Autodesk Fusion 360 part; units mm, degrees
sketch "Sketch1" plane through (0, 0, 0) normal (0, 1, 0) x (1, 0, 0)
  line L0 (16, 0) -> (16, 35)
  line L1 (28.7, 0) -> (28.7, 35)
  line L2 (16, 35) -> (11, 35)
  line L3 (11, 35) -> (11, 0)
  line L4 (16, 0) -> (28.7, 0)
  line L5 (28.7, 35) -> (33.7, 35)
  line L6 (33.7, 35) -> (33.7, 0)
  line L7 (33.7, 0) -> (63.7, 0)
  line L8 (63.7, 0) -> (63.7, -10)
  line L9 (11, 0) -> (-19, 0)
  line L10 (-19, 0) -> (-19, -10)
  line L11 (-19, -10) -> (63.7, -10)
  dimension "d2" = 12.7
  dimension "d3" = 5
  dimension "d4" = 5
  dimension "d5" = 30
  dimension "d6" = 10
  dimension "d7" = 30
  dimension "d8" = 10
  dimension "d16" = 35
extrude "Extrude1" add sketch "Sketch1" along normal blind 35
sketch "Sketch2" plane through (33.7, 0, 0) normal (1, 0, 0) x (0, 0, -1)
  line L0 (0, 0) -> (35, 0)
  line L1 (35, 0) -> (35, 35)
  line L2 (35, 35) -> (0, 35)
  line L3 (0, 35) -> (0, 0)
  circle A0 centre (17.9261, 17.0739) radius 2.25
  line L4 (0, 35) -> (16.3351, 18.6649)
  line L5 (19.5171, 15.4829) -> (35, 0)
  line L6 (35, 35) -> (19.0329, 19.0329)
  line L7 (15.9671, 15.9671) -> (0, 0)
  dimension "d11" = 4.5
extrude "Extrude2" cut sketch "Sketch2" against normal blind 59 contours A0
ref_plane "WorkPlane1" through (22.35, 17.5, -12.5) normal (0, 1, 0) x (0, 0, 1)
sketch "Sketch3" plane through (0, 17.5, 0) normal (0, 1, 0) x (1, 0, 0)
  line L0 (-20, 0) -> (5, 0)
  line L1 (5, 0) -> (5, -10)
  line L2 (5, -10) -> (-20, -10)
  line L3 (-20, -10) -> (-20, 0)
  line L4 (44, 0) -> (44.05, 0)
  line L5 (33.7, 0) -> (33.7, 35)
  dimension "d14" = 25
sketch "Sketch4" plane through (11, 0, 0) normal (-1, 0, 0) x (0, 0, 1)
  circle A0 centre (-17.9261, 17.0739) radius 2.25 construction
  line L0 (-35, 0) -> (0, 0)
  line L1 (0, 0) -> (0, 35)
  line L2 (0, 35) -> (-35, 35)
  line L3 (-35, 35) -> (-35, 0)
  line L4 (-15.8332, 13.4489) -> (-13.7403, 17.0739)
  line L5 (-13.7403, 17.0739) -> (-15.8332, 20.6989)
  line L6 (-15.8332, 20.6989) -> (-20.019, 20.6989)
  line L7 (-20.019, 20.6989) -> (-22.1119, 17.0739)
  line L8 (-22.1119, 17.0739) -> (-20.019, 13.4489)
  line L9 (-20.019, 13.4489) -> (-15.8332, 13.4489)
  point P0 (-17.9261, 17.0739)
  dimension "d18" = 7.25
extrude "Extrude3" cut sketch "Sketch4" against normal blind 3 contours L4 L5 L6 L7 L8 L9
chamfer "Chamfer1" distance 5 angle 45 4 edges at (63.7, 0, 5) (63.7, 35, 5) (-19, 35, 5) (-19, 0, 5)
sketch "Sketch5" plane through (33.7, 0, 0) normal (1, 0, 0) x (0, 0, -1)
  circle A0 centre (17.9261, 17.0739) radius 2.25
  line L0 (0, 0) -> (35, 0)
  line L1 (35, 0) -> (35, 35)
  line L2 (35, 35) -> (0, 35)
  circle A1 centre (17.9261, 17.0739) radius 2.25
  circle A2 centre (17.9261, 17.0739) radius 3.75
  line L3 (0, 35) -> (0, 0)
  dimension "d24" = 7.5
extrude "Extrude4" cut sketch "Sketch5" against normal blind 3.7 contours A2
extrude "Extrude5" cut 1 faces at (14, 18.6077, -15.1575) along direction (1, 0, 0) blind 0.037
extrude "Extrude6" cut 1 faces at (30, 16.7758, -21.1538) along direction (-1, 0, 0) blind 0.663
chamfer "Chamfer2" distance 4 distance2 10 1 edges at (11, 17.5, -35) measured on face at (14.3333, 11.6667, -35)
chamfer "Chamfer2" distance 10 distance2 4 1 edges at (33.7, 17.5, -35) measured on face at (33.7, 30.2711, -17.5486)
extrude "Extrude7" add 1 faces at (14.037, 18.6077, -15.1575) along direction (-1, 0, 0) blind 0.5
extrude "Extrude8" add 1 faces at (29.337, 16.7758, -21.1538) along direction (1, 0, 0) blind 2
extrude "Extrude9" cut 1 faces at (13.537, 18.6077, -15.1575) along direction (1, 0, 0) blind 0.5
extrude "Extrude10" add 1 faces at (31.337, 16.7758, -21.1538) along direction (1, 0, 0) blind 0.5
fillet "Fillet1" radius 10 2 edges at (33.7, 17.5, 0) (11, 17.5, 0)
equation "d5 = d7"
Geometry check sheet. Reference: the model listing, model coordinates, mm. A direction names the side the tool comes from. Coordinates: 2 decimals unless noted, no trailing zeros. Order: outer loops, then holes, each group sorted by start corner. A loop starts at its lowest first (then second) coordinate and runs counter-clockwise, first axis right, second up. Notation, with made-up numbers: M 1,-22 L 14,-22 A25 ccw 14,-8 Z; hole C -23.5,-31 d6. An arc over 180 degrees is marked long. Use CSV: the item, a comma, the result in double quotes.
Item 1: Tool access check on faces 4 (the flat face through (31.837, 15, -20)), 5 (the flat face through (12, 20.699, -18)), 6 (the flat face through (22, 17, 0)), 7 (the flat face through (-9, 17, 0)), 8 (the flat face through (33.7, 21, -18)). Record the directions out of +Z, -Z, +X, -X, +Y, -Y that give a thin tool (end or side, any length) a straight path to the whole face; none if there is none.
Returned:
face 4,"+X"
face 5,"-X"
face 6,"-Z, +Y, -Y"
face 7,"-Z, -X, +Y, -Y"
face 8,"-Z, +X, +Y, -Y"
Item 2: Mould release check, pull along Y, two halves, no side actions. Record for faces 1 (the flat face through (22, 35, 2)), 2 (the flat face through (28.7, 21, -17)), 3 (the flat face through (12.5, 18.86, -14.77)): pulls with the +Y half, pulls with the -Y half, needs draft (parallel to the pull), parting line crosses it, or undercut.
Returned:
face 1,"pulls with the +Y half"
face 2,"needs draft"
face 3,"undercut"
Item 3: Cross-section at B-B on y = 18.5. Give the number of separate pieces and of enclosed holes in the cut face, then the cut area to 3 significant figures.
Returned:
separate pieces,"3"
enclosed holes,"0"
area,"1,130 mm2"
Item 4: Cross-section at A-A on z = -27.5. Record the cut outline in (x, y).
Returned:
outline,"M 12,0 L 16,0 L 16,35 L 12,35 Z; M 28.7,0 L 32.7,0 L 32.7,35 L 28.7,35 Z"
Item 5: Gauge pin test, flat ends, axial feed: pin 1 Ø4 at (y, z) = (17.07, -17.93) entering from +X; pin 2 Ø12 at (y, z) = (17.07, -17.93) entering from +X; pin 3 Ø16 at (x, y) = (-11.5, 13) entering from -Z; pin 4 Ø12 at (y, z) = (16, -15.5) entering from -X. Record the tip position at first contact, or that the pin passes through.
Returned:
pin 1,"passes through"
pin 2,"stops at x = 33.7"
pin 3,"stops at z = 0"
pin 4,"stops at x = 10.99"
Item 6: Thickness scan on line 1 along X through (y, z) = (24, -24); line 2 along X through (y, z) = (16.5, -15); line 3 along Z through (x, y) = (-6, 21). Record the ranges inside material, lowest first.
Returned:
line 1,"x = 11 to 16, 28.7 to 33.7"
line 2,"x = 14.04 to 16, 28.7 to 31.84"
line 3,"z = 0 to 10"
Item 7: Cross-section at C-C on y = 3. Record the cut outline in (x, z), then the cut area to 3 significant figures.
Returned:
outline,"M -17,0 L 1,0 A10 cw 11,-10 L 11,-25 L 15,-35 L 16,-35 L 16,0 L 28.7,0 L 28.7,-35 L 29.7,-35 L 33.7,-25 L 33.7,-10 A10 cw 43.7,0 L 61.7,0 L 61.7,10 L -17,10 Z"
area,"1,140 mm2"
Item 8: Cross-section at D-D on x = 22. Record the cut outline in (y, z), then the cut area to 3 significant figures.
Returned:
outline,"M 0,0 L 35,0 L 35,10 L 0,10 Z"
area,"350 mm2"
